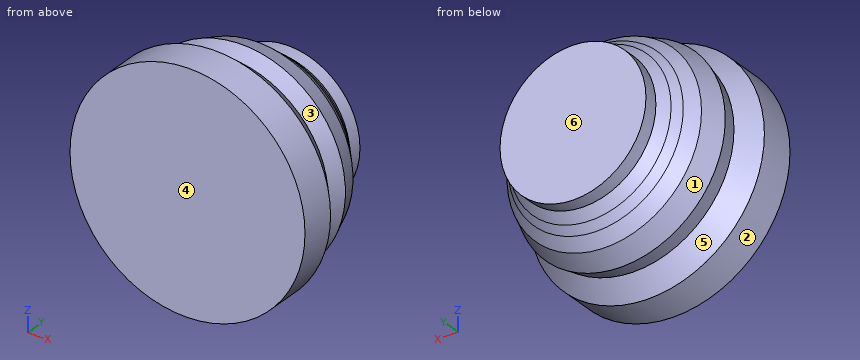
Autodesk Inventor part; units mm, degrees
ref_plane "YZ Plane" through (0, 0, 0) normal (1, 0, 0) x (0, 1, 0)
ref_plane "XZ Plane" through (0, 0, 0) normal (0, 1, 0) x (-1, 0, 0)
ref_plane "XY Plane" through (0, 0, 0) normal (0, 0, 1) x (1, 0, 0)
sketch "Boceto2" plane through (0, 0, 0) normal (0, 0, 1) x (1, 0, 0)
  line L0 (-55.132, 97.6233) -> (57.4508, 97.6233) construction
  line L1 (57.4508, 97.6233) -> (57.4508, -13.0832) construction
  line L2 (57.4508, -13.0832) -> (-55.132, -13.0832) construction
  line L3 (-55.132, -13.0832) -> (-55.132, 97.6233) construction
  line L4 (0, 0) -> (0, 27.5828)
  line L5 (0, 27.5828) -> (0, 0)
  line L6 (-22.8755, 0.7881) -> (-22.8755, 7.0927)
  line L7 (-22.8755, 7.0927) -> (-19.7232, 11.0331)
  line L8 (-19.7232, 11.0331) -> (-20.5113, 14.5795)
  line L9 (-20.5113, 14.5795) -> (-18.9351, 18.9139)
  line L10 (-18.9351, 18.9139) -> (-17.0437, 21.2782)
  line L11 (-17.0437, 21.2782) -> (-15.7828, 22.8543)
  line L12 (-15.7828, 22.8543) -> (-14.2066, 24.8245)
  line L13 (-14.2066, 24.8245) -> (-14.2066, 27.5828)
  line L14 (-14.2066, 27.5828) -> (-12, 27.5828)
  line L15 (0, 27.5828) -> (-12, 27.5828)
  line L16 (-14.2066, 27.5828) -> (-12, 27.5828)
  line L17 (0, 0) -> (-22.8755, 0)
  line L18 (-22.8755, 0) -> (-22.8755, 0.7881)
  dimension "d18" = 12
revolve "Revolución1" add sketch "Boceto2" angle 360 about axis through (0, 0, 0) along (0, 1, 0)
properties part number "KINGHT BASE  medieum 1.0"
The listing builds one solid part. Answer for the finished solid, in the listing's coordinates (mm). Face numbers are marked on the shaded views. A direction names the side the tool comes from. Give positions to 0.01 mm unless a question says otherwise; leave off trailing zeros. Order: outer loops, then holes, each group sorted by start corner. A loop starts at its lowest first (then second) coordinate and runs counter-clockwise, first axis right, second up.
1) Find section A-A on z = 0. Write down the section's boundary in (x, y).
Reported:
outline: (-22.88, 0) - (22.88, 0) - (22.88, 7.09) - (19.72, 11.03) - (20.51, 14.58) - (18.94, 18.91) - (17.04, 21.28) - (15.78, 22.85) - (14.21, 24.82) - (14.21, 27.58) - (-14.21, 27.58) - (-14.21, 24.82) - (-15.78, 22.85) - (-17.04, 21.28) - (-18.94, 18.91) - (-20.51, 14.58) - (-19.72, 11.03) - (-22.88, 7.09) - close
2) Find section C-C on y = 14. Write down the section's boundary in (x, z).
Reported:
outline: circle Ø40.77 at (0, 0)
3) For the marked faces 5 and 6, determine the directions among +Z, -Z, +X, -X, +Y, -Y from which every point of the face is accessible in a straight line to the end or side of a thin tool.
Reported:
face 5: none
face 6: +Z, -Z, +X, -X, +Y
4) Consider line 1 along X through (y, z) = (10.25, -8.5); line 2 along X through (y, z) = (2.5, 12.5); line 3 along Y through (x, z) = (-5, -21). Determine where each line is inside the solid, lowest interval first.
Reported:
line 1: x = -18.49 to 18.49
line 2: x = -19.16 to 19.16
line 3: y = 0 to 8.7
5) Given P1, Ø6, axis at y = 20.5, z = 13, coming from the -X side; P2, Ø8, axis at y = 9.5, z = 13.5, coming from the +X side; P3, Ø8, axis at x = 5.5, y = 11.5, coming from the -Z side, each flat-ended and moving along its own axis, determine where each tip first touches the part or whether it passes through.
Reported:
P1: stops at x = -15.79
P2: stops at x = 20.42
P3: stops at z = -21.99
6) Find section B-B on x = 0. Write down the section's boundary in (y, z).
Reported:
outline: (0, -22.88) - (7.09, -22.88) - (11.03, -19.72) - (14.58, -20.51) - (18.91, -18.94) - (21.28, -17.04) - (22.85, -15.78) - (24.82, -14.21) - (27.58, -14.21) - (27.58, 14.21) - (24.82, 14.21) - (22.85, 15.78) - (21.28, 17.04) - (18.91, 18.94) - (14.58, 20.51) - (11.03, 19.72) - (7.09, 22.88) - (0, 22.88) - close
7) Find section D-D on y = 23.5. Write down the section's boundary in (x, z).
Reported:
outline: circle Ø30.53 at (0, 0)
8) Determine the mould class of the marked faces 1, 2, 3 and 4 for opening direction Y: pulls with the +Y half, pulls with the -Y half, needs draft (parallel to the pull), parting line crosses it, or undercut.
Reported:
face 1: pulls with the +Y half
face 2: needs draft
face 3: undercut
face 4: pulls with the -Y half
